from build123d import *

# Parameters (mm, degrees)
BOTTOM_LEVEL_DEPTH = 5
MID_LEVEL_DEPTH    = 35
GUARD_RAIL_DEPTH   = 100
ROUNDING_R         = 5


with BuildPart() as part:
    # Sketch1 → Bottom level (new body)
    with BuildSketch(Plane(origin=(0, 0, 0), x_dir=(1, 0, 0), z_dir=(0, 1, 0))):
        with BuildLine():
            Line((481, 481), (531, 481))
            Line((531, 481), (531, 456))
            Line((531, 456), (481, 456))
            ThreePointArc((481, 456), (158.559307779, 322.440692221), (25, 0))
            Line((25, 0), (0, 0))
            ThreePointArc((0, 0), (140.881638249, 340.118361751), (481, 481))
        make_face()
    extrude(amount=BOTTOM_LEVEL_DEPTH)

    # Sketch2 → Mid level (add)
    with BuildSketch(Plane(origin=(0, 5, 0), x_dir=(1, 0, 0), z_dir=(0, 1, 0))):
        with BuildLine():
            Line((481, 456), (531, 456))
            Line((531, 456), (531, 471))
            Line((531, 471), (481, 471))
            ThreePointArc((481, 471), (147.952706061, 333.047293939), (10, 0))
            Line((10, 0), (25, 0))
            ThreePointArc((25, 0), (158.559307779, 322.440692221), (481, 456))
        make_face()
    extrude(amount=MID_LEVEL_DEPTH)

    # Sketch3 → Guard rail (add)
    with BuildSketch(Plane(origin=(0, 40, 0), x_dir=(1, 0, 0), z_dir=(0, 1, 0))):
        with BuildLine():
            Line((481, 456), (531, 456))
            Line((531, 456), (531, 461))
            Line((531, 461), (481, 461))
            ThreePointArc((481, 461), (155.023773873, 325.976226127), (20, 0))
            Line((20, 0), (25, 0))
            ThreePointArc((25, 0), (158.559307779, 322.440692221), (481, 456))
        make_face()
    extrude(amount=GUARD_RAIL_DEPTH)

    # Rounding
    rounding_edges = [part.edges().sort_by_distance(p)[0] for p in [
        (506, 40, -461),
        (506, 40, -471),
        (506, 5, -471),
        (155.023773873, 40, -325.976226127),
        (147.952706061, 40, -333.047293939),
        (147.952706061, 5, -333.047293939),
    ]]
    fillet(rounding_edges, radius=ROUNDING_R - 0.0001)  # a hair under: the kernel refuses the full size


solid = part.part
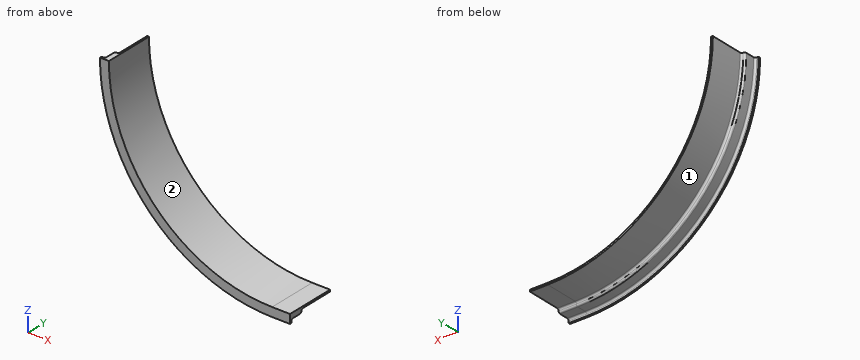
Read the model definition and answer for the solid it produces. Units are mm, in the model's axes. Face numbers are marked on the shaded views. A direction names the side the tool comes from. Round coordinates to 2 decimals unless told otherwise and drop trailing zeros. Order: outer loops, then holes, each group sorted by start corner. A loop starts at its lowest first (then second) coordinate and runs counter-clockwise, first axis right, second up.
1) Flat-ended cylindrical pins translate along their axes: pin 1 (15 mm diameter, centred on x = 509, y = 82.5, fed in from -Z); pin 2 (5 mm diameter, centred on y = 22.5, z = -65.5, fed in from +X); pin 3 (25 mm diameter, centred on x = 513.5, y = 103, fed in from +Z). Find the tip coordinate at first contact, or state that the pin passes through.
2) For the marked faces 1 and 2, determine the directions among +Z, -Z, +X, -X, +Y, -Y from which every point of the face is accessible in a straight line to the end or side of a thin tool.
3) The part is cut by section A-A on y = 28.5. Write down the section's boundary in (x, z), plus the area to 3 significant figures.
4) The part is cut by section B-B on y = 72. Write down the section's boundary in (x, z), plus the area to 3 significant figures.
5) Straight lines are drawn through the part: L1, parallel to X at y = 74.5, z = -304.5; L2, parallel to X at y = 36, z = -232.5; L3, parallel to Z at x = 243, y = 16. For each, find the intervals that lie inside material, in ascending order.
Resolved:
1. pin 1: stops at z = -461
1. pin 2: stops at x = 30.1
1. pin 3: stops at z = -456
2. face 1: -Z, -X, +Y
2. face 2: +Z, +X, +Y, -Y
3. outline: (10, 0) arc R471 ccw to (481, -471) - (531, -471) - (531, -456) - (481, -456) arc R456 cw to (25, 0) - close
3. area: 11,700 mm2
4. outline: (20, 0) arc R461 ccw to (481, -461) - (531, -461) - (531, -456) - (481, -456) arc R456 cw to (25, 0) - close
4. area: 3,850 mm2
5. L1: x = 134.88 to 141.57
5. L2: x = 71.5 to 88.72
5. L3: z = -406.44 to -388.96
